Input: part model. Units: mm. Frame: model coordinates. A direction names the side the tool comes from. Round coordinates to 2 decimals unless told otherwise and drop trailing zeros. Loops run counter-clockwise (first coordinate to the right, second up) from the corner with the lowest first, then second, coordinate; pieces in that order, holes last. Notation, with made-up numbers: (69.25, 84) -> (100.25, 84) arc R11 ccw to (100.25, 101) -> close; hole circle Ø10 at (49, 41). An arc over 180 degrees is marked (long way). Answer as a JSON object with one key per item and string values.
Autodesk Inventor part; units mm, degrees
ref_plane "Work Plane1" through (0, -10, 0) normal (0, 0, -1) x (-1, 0, 0)
ref_plane "YZ Plane" through (0, 0, 0) normal (1, 0, 0) x (0, 1, 0)
ref_plane "XZ Plane" through (0, 0, 0) normal (0, 1, 0) x (-1, 0, 0)
sketch "Sketch1" plane through (0, 0, 0) normal (1, 0, 0) x (0, 1, 0)
  line L0 (10, 10) -> (-10, 10)
  line L1 (-10, 10) -> (-10, -10)
  line L2 (-10, -10) -> (10, -10)
  line L3 (10, -10) -> (10, 10)
  line L4 (10, 10) -> (-10, -10) construction
  line L5 (-10, 10) -> (10, -10) construction
  circle A0 centre (0, 0) radius 14.1421
  circle A1 centre (0, 0) radius 20
  dimension "d0" = 20
  dimension "d1" = 20
  dimension "d2" = 40
extrude "Extrusion1" add sketch "Sketch1" along normal blind 10 contours A0 L3 | L0 A0 | L1 A0 | A0 L2 | A1
ref_plane "Work Plane1" through (0, -10, 0) normal (0, 0, -1) x (-1, 0, 0)
sketch "Sketch2" plane through (0, -10, 0) normal (0, 0, -1) x (-1, 0, 0)
  line L0 (0, 30) -> (-10, 30)
  line L1 (0, 30) -> (-5, 30)
  line L2 (-5, 30) -> (-2, 30)
  line L3 (-5, 30) -> (-8, 30)
  line L4 (-8, 30) -> (-8, 29)
  line L5 (-8, 29) -> (-3, 29)
  line L6 (-8, 29) -> (-2, 29)
  line L7 (-2, 29) -> (-2, 30)
  line L8 (-2, 30) -> (-8, 30)
  line L9 (-8, 30) -> (-8, 29)
  line L10 (2, 10) -> (-12, 10)
  point P0 (0, 10)
  point P1 (-2.5, 28)
  dimension "d5" = 3
  dimension "d6" = 3
  dimension "d7" = 1
revolve "Revolution1" cut sketch "Sketch2" angle 360 about axis through (-10, 0, 0) along (1, 0, 0)
sketch "Sketch4" plane through (8, 0, 0) normal (-1, 0, 0) x (0, 0, 1)
  line L0 (0, -19.0057) -> (0, -20.5057)
  circle A0 centre (0, -20.5057) radius 1.5
  point P0 (0, 0)
  dimension "d12" = 1.5
extrude "Extrusion3" cut sketch "Sketch4" against normal blind 10
properties part number "antenna_rad" material "PET Plastic"
1) Section A-A, the plane y = 0. Output: boundary loops of the cut face in (x, z).
Output:
{"outline": "(0, -20) -> (2, -20) -> (2, -19) -> (8, -19) -> (8, -20) -> (10, -20) -> (10, -10) -> (0, -10) -> close; (0, 10) -> (10, 10) -> (10, 20) -> (8, 20) -> (8, 19) -> (2, 19) -> (2, 20) -> (0, 20) -> close"}
2) Draft query along Z for faces 1 (the face through (0.986, -4.336, 19.524)), 2 (the face through (5, 10, 0)), 3 (the face through (10, 0, -13)), 4 (the face through (5, 0, 10)). Return one class per face: +Z half, -Z half, draft (parallel to the pull), parting line (faces both ways), or undercut.
Output:
{"face 1": "parting line", "face 2": "undercut", "face 3": "draft", "face 4": "undercut"}
3) Ray query, probe 1 along Y at (x, z) = (3.5, 4.5); probe 2 along Z at (x, y) = (4.5, -2); probe 3 along Z at (x, y) = (2.75, -3). Return the intervals inside material, ascending.
Output:
{"probe 1": "y = -18.46 to -10, 10 to 18.46", "probe 2": "z = -18.89 to -10, 10 to 18.89", "probe 3": "z = -18.76 to -10, 10 to 18.76"}
4) Section D-D, the plane z = 10.5. Output: boundary loops of the cut face in (x, y).
Output:
{"outline": "(0, -17.02) -> (2, -17.02) -> (2, -15.84) -> (8, -15.84) -> (8, -17.02) -> (10, -17.02) -> (10, 17.02) -> (8, 17.02) -> (8, 15.84) -> (2, 15.84) -> (2, 17.02) -> (0, 17.02) -> close"}
5) Reachability of faces 5 (the face through (8.986, -19.006, 0.025)), 6 (the face through (5, -10, 0)), 7 (the face through (4.958, 8.767, 16.856)) from +Z, -Z, +X, -X, +Y, -Y: full face, straight path, thin tool, end or side. Return the list, or none.
Output:
{"face 5": "+X, -Y", "face 6": "+X, -X", "face 7": "none"}
6) Section C-C, the plane z = -5. Output: boundary loops of the cut face in (x, y), plus the area to 3 significant figures.
Output:
{"outline": "(0, -19.36) -> (2, -19.36) -> (2, -18.33) -> (8, -18.33) -> (8, -19.36) -> (10, -19.36) -> (10, -10) -> (0, -10) -> close; (0, 10) -> (10, 10) -> (10, 19.36) -> (8, 19.36) -> (8, 18.33) -> (2, 18.33) -> (2, 19.36) -> (0, 19.36) -> close", "area": "175 mm^2"}
7) Section B-B, the plane x = 2.5. Output: boundary loops of the cut face in (y, z), plus the area to 3 significant figures.
Output:
{"outline": "circle Ø38 at (0, 0); hole (-10, -10) -> (10, -10) -> (10, 10) -> (-10, 10) -> close", "area": "734 mm^2"}
8) Contact query for flat-ended pins moving along their axis: P1, Ø4, axis at x = 2.5, z = 9.5, coming from the -Y side; P2, Ø20, axis at y = 6.5, z = 2.5, coming from the -X side; P3, Ø1, axis at x = 4, z = 13.5, coming from the -Y side; P4, Ø3, axis at x = 3, y = 12, coming from the +Z side. Output: stop coordinate, or through.
Output:
{"P1": "stops at y = -18.51", "P2": "stops at x = 0", "P3": "stops at y = -13.86", "P4": "stops at z = 16.78"}
